from build123d import *

# Parameters (mm, degrees)
SKETCH1_R           = 10
BOSS_EXTRUDE1_DEPTH = 25
SKETCH2_R           = 4
CUT_EXTRUDE1_DEPTH  = 26
FILLET1_R           = 2


with BuildPart() as part:
    # Sketch1 → Boss-Extrude1 (new body)
    with BuildSketch(Plane(origin=(0, 0, 0), x_dir=(0, 0, -1), z_dir=(1, 0, 0))):
        Circle(SKETCH1_R)
    extrude(amount=BOSS_EXTRUDE1_DEPTH)

    # Sketch2 → Cut-Extrude1 (cut, through all)
    with BuildSketch(Plane(origin=(25, 0, 0), x_dir=(0, 0, -1), z_dir=(1, 0, 0))):
        Circle(SKETCH2_R)
    extrude(amount=-CUT_EXTRUDE1_DEPTH, mode=Mode.SUBTRACT)

    # Fillet1
    fillet1_edges = [part.edges().sort_by_distance(p)[0] for p in [
        (0, 0, 10),
        (25, 0, 10),
    ]]
    fillet(fillet1_edges, radius=FILLET1_R)


solid = part.part
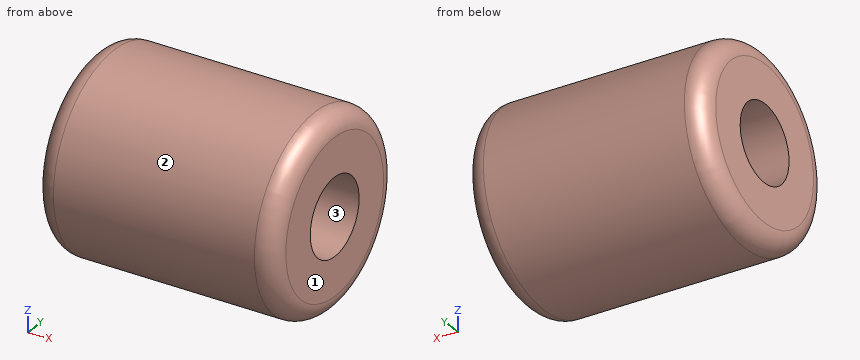
Source: CAD feature listing. Evaluate the final solid. Frame: model axes, mm. Face numbers are marked on the shaded views. Give positions to 0.01 mm unless a question says otherwise; leave off trailing zeros. Write each loop counter-clockwise with the first axis right and the second up, starting at its lowest first coordinate (ties: lowest second). Pieces come first, ordered by that corner, then holes. Notation, with made-up numbers: (62.5, 11) - (74.5, 11) arc R4 cw to (74.5, 15) - close; hole circle Ø1 at (-9.5, -38.5). An arc over 180 degrees is marked (long way). Write item = value, one per line. Start each with the question number.
Q1. Cut plane C-C, the plane x = 6. Return loops of the section in (y, z).
Q2. Cut plane A-A, the plane z = 0. Return loops of the section in (x, y).
Q3. Material intervals for probe 1 along Y at (x, z) = (7, 0); probe 2 along Y at (x, z) = (15, -2); probe 3 along Z at (x, y) = (14, 3), sorted ascending.
Q4. Draft query along Z for the marked faces 1, 2 and 3. Return one class per face: +Z half, -Z half, draft (parallel to the pull), parting line (faces both ways), or undercut.
Q5. Pin query (flat end, axial travel): pin 1 Ø4 at (x, z) = (3.5, 3.5) entering from +Y; pin 2 Ø1.5 at (x, y) = (10.5, -5.5) entering from -Z; pin 3 Ø5 at (x, z) = (7, 3) entering from -Y. Return the tip coordinate at first contact, or that it passes through.
Computed values:
q1.outline = circle Ø20 at (0, 0); hole circle Ø8 at (0, 0)
q2.outline = (0, -8) arc R2 ccw to (2, -10) - (23, -10) arc R2 ccw to (25, -8) - (25, -4) - (0, -4) - close; (0, 4) - (25, 4) - (25, 8) arc R2 ccw to (23, 10) - (2, 10) arc R2 ccw to (0, 8) - close
q3.probe_1 = -10 to -4, 4 to 10
q3.probe_2 = -9.8 to -3.46, 3.46 to 9.8
q3.probe_3 = -9.54 to -2.65, 2.65 to 9.54
q4.face_1 = draft
q4.face_2 = parting line
q4.face_3 = undercut
q5.pin_1 = 9.89
q5.pin_2 = -8.8
q5.pin_3 = -9.99
